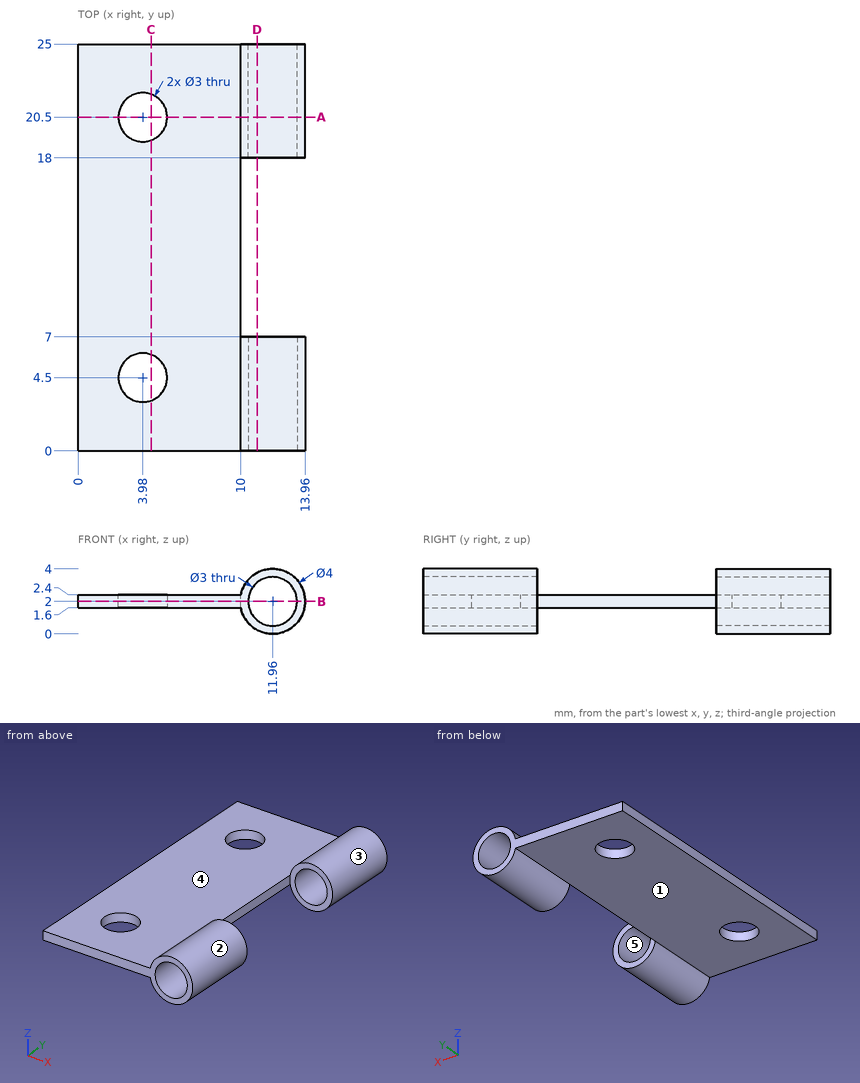
Study the drawing (mm; zero at the part's minimum x, y, z) and answer. A direction names the side the tool comes from. Give positions to 0.01 mm unless a question says otherwise; leave off trailing zeros. Loops run counter-clockwise (first coordinate to the right, second up) from the corner with the lowest first, then second, coordinate; pieces in that order, holes last. Notation, with made-up numbers: M 3,73.5 L 10,73.5 A23 ccw 10,96.5 Z; hole C 12.5,-6.75 d4. An arc over 180 degrees is marked long. One line per item, written item: value. Start each with the question number.
1. Find section C-C (x = 4.5). Give the vertices of the cut face in (y, z), and give its area (3 significant figures).
2. Find section A-A (y = 20.5). Give the vertices of the cut face in (x, z).
3. Determine the mould class of the marked faces 3, 4 and 5 for opening direction Z: released by +Z, released by -Z, zero draft, split by the parting line, or undercut.
4. Find the intervals of material crossed by probe 1 along X at (y, z) = (22.25, 2); probe 2 along X at (y, z) = (5.5, 2); probe 3 along Z at (x, y) = (4.5, 12), in increasing order.
5. Which of the six approach directions +Z, -Z, +X, -X, +Y, -Y give full straight-line access (tool end or side, diameter ignored) to the marked faces 1 and 2?
6. Find section B-B (z = 2). Give the vertices of the cut face in (x, y).
7. Find section D-D (x = 11). Give the vertices of the cut face in (y, z) (1 decimal).
8. Each of these flat-tipped pins is pushed along its axis until it touches: P1, Ø5, axis at x = 3.98, y = 4.5, coming from the -Z side; P2, Ø3, axis at x = 5.5, y = 6.5, coming from the +Z side; P3, Ø2, axis at y = 12, z = 2.5, coming from the +X side. Where does it stop, or does it pass through?
Reported:
1. outline: M 0,1.6 L 3.09,1.6 L 3.09,2.4 L 0,2.4 Z; M 5.91,1.6 L 19.09,1.6 L 19.09,2.4 L 5.91,2.4 Z; M 21.91,1.6 L 25,1.6 L 25,2.4 L 21.91,2.4 Z
1. area: 15.5 mm²
2. outline: M 0,1.6 L 2.48,1.6 L 2.48,2.4 L 0,2.4 Z; M 5.48,1.6 L 10,1.6 A2 ccw long 10,2.4 L 5.48,2.4 Z; hole C 11.96,2 d3
3. face 3: split by the parting line
3. face 4: released by +Z
3. face 5: undercut
4. probe 1: x = 0 to 10.46, 13.46 to 13.96
4. probe 2: x = 0 to 2.86, 5.1 to 10.46, 13.46 to 13.96
4. probe 3: z = 1.6 to 2.4
5. face 1: -Z, -X, +Y, -Y
5. face 2: +Y, -Y
6. outline: M 0,0 L 10.46,0 L 10.46,7 L 10,7 L 10,18 L 10.46,18 L 10.46,25 L 0,25 Z; M 13.46,0 L 13.96,0 L 13.96,7 L 13.46,7 Z; M 13.46,18 L 13.96,18 L 13.96,25 L 13.46,25 Z; hole C 3.98,4.5 d3; hole C 3.98,20.5 d3
7. outline: M 0,0.2 L 7,0.2 L 7,0.8 L 0,0.8 Z; M 0,3.2 L 7,3.2 L 7,3.8 L 0,3.8 Z; M 18,0.2 L 25,0.2 L 25,0.8 L 18,0.8 Z; M 18,3.2 L 25,3.2 L 25,3.8 L 18,3.8 Z
8. P1: stops at z = 1.6
8. P2: stops at z = 2.4
8. P3: stops at x = 10
